Geometry: final body of the model. Coordinates: model frame, mm. A direction names the side the tool comes from. Round coordinates to 2 decimals unless told otherwise and drop trailing zeros. Order: outer loops, then holes, each group sorted by start corner. A loop starts at its lowest first (then second) coordinate and runs counter-clockwise, first axis right, second up. Notation, with made-up numbers: M 60.5,7 L 109.5,7 A25 cw 109.5,27 Z; hole C 68,76.5 d6. An arc over 180 degrees is marked long. Put each result on its own line as item: value. Start each with the question number.
1) Access query for faces 1 (the flat face through (20, 18, 150)), 2 (the cylindrical face through (29.54, 21, 84.09)). Directions: +Z, -Z, +X, -X, +Y, -Y. A direction counts if a zero-diameter tool reaches every point of the face in a straight line with its end or side. Return the directions, or none.
2) Section B-B, the plane x = 20. Return loops of the section in (y, z), then the cut area to 3 significant figures.
3) First-contact query: P1, Ø8, axis at y = 30.5, z = 27, coming from the -X side; P2, Ø10, axis at x = 117.5, y = 29, coming from the +Z side; P3, Ø6, axis at y = 13, z = 61, coming from the +X side. Flat tips, straight axial feed; report the tip coordinate or a pass-through.
4) Section C-C, the plane z = 12.5. Return loops of the section in (x, y), then the cut area to 3 significant figures.
5) Draft query along X for faces 3 (the flat face through (0, 18, 10)), 4 (the flat face through (157, 18, 20)), 5 (the cylindrical face through (290, 18, 10)). Return one class per face: pulls with the +X half, pulls with the -X half, needs draft (parallel to the pull), parting line crosses it, or undercut.
6) Section D-D, the plane x = 293. Return loops of the section in (y, z), then the cut area to 3 significant figures.
7) Section A-A, the plane y = 18. Return loops of the section in (x, z), then the cut area to 3 significant figures.
8) Material intervals for probe 1 along Y at (x, z) = (300, 15.5); probe 2 along Z at (x, y) = (46, 10); probe 3 along Y at (x, z) = (19, 42), sorted ascending. Write a range as [from, to].
from build123d import *

# Parameters (mm, degrees)
ESQUISSE1_R        = 10
BOSS_EXTRU_1_DEPTH = 20
ESQUISSE2_R        = 10
BOSS_EXTRU_2_DEPTH = 130


with BuildPart() as part:
    # Esquisse1 → Boss.-Extru.1 (new body)
    with BuildSketch(Plane.XY):
        with BuildLine():
            Line((0, 0), (300, 0))
            ThreePointArc((300, 0), (318, 18), (300, 36))
            Line((300, 36), (0, 36))
            Line((0, 36), (0, 0))
        make_face()
        with Locations((300, 18)):
            Circle(ESQUISSE1_R, mode=Mode.SUBTRACT)
    extrude(amount=BOSS_EXTRU_1_DEPTH)

    # Esquisse2 → Boss.-Extru.2 (add)
    with BuildSketch(Plane.XY.offset(20)):
        with Locations((20, 18)):
            Circle(ESQUISSE2_R)
    extrude(amount=BOSS_EXTRU_2_DEPTH)


solid = part.part
Result sheet:
1. face 1: +Z, +X, -X, +Y, -Y
1. face 2: +Z
2. outline: M 0,0 L 36,0 L 36,20 L 28,20 L 28,150 L 8,150 L 8,20 L 0,20 Z
2. area: 3,320 mm2
3. P1: stops at x = 14.73
3. P2: stops at z = 20
3. P3: stops at x = 29.8
4. outline: M 0,0 L 300,0 A18 ccw 300,36 L 0,36 Z; hole C 300,18 d20
4. area: 11,000 mm2
5. face 3: pulls with the -X half
5. face 4: needs draft
5. face 5: undercut
6. outline: M 0,0 L 10.86,0 L 10.86,20 L 0,20 Z; M 25.14,0 L 36,0 L 36,20 L 25.14,20 Z
6. area: 434 mm2
7. outline: M 0,0 L 290,0 L 290,20 L 30,20 L 30,150 L 10,150 L 10,20 L 0,20 Z; M 310,0 L 318,0 L 318,20 L 310,20 Z
7. area: 8,560 mm2
8. probe 1: y = [0, 8], [28, 36]
8. probe 2: z = [0, 20]
8. probe 3: y = [8.05, 27.95]
